Could you check a few things on this model? Use its own coordinates, in mm. A direction names the side the tool comes from. Give positions to 0.01 mm unless a question says otherwise; leave off trailing zeros. Write each loop counter-clockwise with the first axis right and the second up, starting at its lowest first coordinate (ties: lowest second). Pieces come first, ordered by that corner, then holes. Notation, with made-up numbers: (48, -38.5) -> (72, -38.5) arc R24 cw to (72, -5.5) -> close; hole circle Ø1 at (19, 79.5). An arc over 180 degrees is marked (long way). Write item = value, one per line. Start each with the question number.
```python
from build123d import *

# Parameters (mm, degrees)
F0_W     = 50.8
F0_H     = 25.4
F0_W_2   = 44.45
F0_H_2   = 19.05
F1_DEPTH = 463.55
F2_R     = 2.5781
F3_DEPTH = 50.801
F4_R     = 4.7625
F5_DEPTH = 25.401


with BuildPart() as f1:
    # F0 (on Front) → F1 (new body)
    with BuildSketch(Plane.XZ):
        with Locations((-6.57482, 3.593568)):
            Rectangle(F0_W, F0_H)
        with Locations((-6.57482, 3.593568)):
            Rectangle(F0_W_2, F0_H_2, mode=Mode.SUBTRACT)
    extrude(amount=F1_DEPTH)

    # F2 (on face) → F3 (cut, through all)
    with BuildSketch(Plane(origin=(-31.97482, 0, 0), x_dir=(0, -1, 0), z_dir=(-1, 0, 0))):
        with Locations((12.7, 3.593568)):
            Circle(F2_R)
        with Locations((38.1, 3.593568)):
            Circle(F2_R)
        with Locations((63.5, 3.593568)):
            Circle(F2_R)
        with Locations((400.05, 3.593568)):
            Circle(F2_R)
        with Locations((425.45, 3.593568)):
            Circle(F2_R)
        with Locations((450.85, 3.593568)):
            Circle(F2_R)
    extrude(amount=-F3_DEPTH, mode=Mode.SUBTRACT)

    # F4 (on face) → F5 (cut, through all)
    with BuildSketch(Plane.XY.offset(16.293568)):
        with Locations((-6.57482, -438.15)):
            Circle(F4_R)
        with Locations((-6.57482, -25.4)):
            Circle(F4_R)
    extrude(amount=-F5_DEPTH, mode=Mode.SUBTRACT)


solid = f1.part
```
(1) Imagine slicing it at B-B (x = 10). Please give me the cut outline in (y, z).
(2) If I drill on line 1 along Y through (x, z) = (-6, 14.75); line 2 along Z through (x, y) = (17.95, -12.7); line 3 along X through (y, z) = (-81, 11.5), over which ranges is the centre line in solid material (lowest first)? Write a range as from..to.
(3) Imagine slicing it at C-C (y = -438.15). Please give me the cut outline in (x, z).
(4) Imagine slicing it at A-A (y = -241.5). Please give me the cut outline in (x, z).
(5) We'd pull the mould along Y, two halves only. Please class faces 3 (the cylindrical face through (-7.195, -20.678, -7.497)), 4 (the flat face through (-31.975, -229, 3)), 5 (the flat face through (-7, -463.55, 14)): released by +Y, released by -Y, zero draft, split by the parting line, or undercut.
(6) On a 3-axis mill with a long thin cutter (end or side, diameter ignored), from which of +Z, -Z, +X, -X, +Y, -Y can I reach the whole of each face in a straight line? I mean faces 1 (the cylindrical face through (-7.6, -442.8, 14.7)), 2 (the flat face through (15.65, -229, 3)). Say none if no direction works.
Answers below:
q1.outline = (-463.55, -9.11) -> (0, -9.11) -> (0, -5.93) -> (-463.55, -5.93) -> close; (-463.55, 13.12) -> (0, 13.12) -> (0, 16.29) -> (-463.55, 16.29) -> close
q2.line_1 = -463.55..-442.88, -433.42..-30.13, -20.67..0
q2.line_2 = -9.11..1.02, 6.17..16.29
q2.line_3 = -31.97..-28.8, 15.65..18.83
q3.outline = (-31.97, -9.11) -> (-11.34, -9.11) -> (-11.34, -5.93) -> (-28.8, -5.93) -> (-28.8, 13.12) -> (-11.34, 13.12) -> (-11.34, 16.29) -> (-31.97, 16.29) -> close; (-1.81, -9.11) -> (18.83, -9.11) -> (18.83, 16.29) -> (-1.81, 16.29) -> (-1.81, 13.12) -> (15.65, 13.12) -> (15.65, -5.93) -> (-1.81, -5.93) -> close
q4.outline = (-31.97, -9.11) -> (18.83, -9.11) -> (18.83, 16.29) -> (-31.97, 16.29) -> close; hole (-28.8, -5.93) -> (15.65, -5.93) -> (15.65, 13.12) -> (-28.8, 13.12) -> close
q5.face_3 = undercut
q5.face_4 = zero draft
q5.face_5 = released by -Y
q6.face_1 = +Z, -Z
q6.face_2 = +Y, -Y
